Build history of the part. All positions in model axes, mm. A direction names the side the tool comes from. Round coordinates to 2 decimals unless told otherwise and drop trailing zeros. Loops run counter-clockwise (first coordinate to the right, second up) from the corner with the lowest first, then second, coordinate; pieces in that order, holes last. Notation, with made-up numbers: M 85.5,0.5 L 127.5,0.5 A12 cw 127.5,10.5 Z; hole C 62,3.5 d9. An arc over 180 degrees is marked long. Write each question's results on one line, items separated by ' | '. Start each with the question number.
```python
from build123d import *
from build123d.topology import SkipClean

# Parameters (mm, degrees)
CUT_EXTRUDE1_DEPTH  = 11
FILLET1_R           = 8
SKETCH3_R           = 3
CUT_EXTRUDE2_DEPTH  = 3
SKETCH4_R           = 5
CUT_EXTRUDE3_DEPTH  = 4.5
SKETCH5_R           = 25
CUT_EXTRUDE4_DEPTH  = 152.297719745
SKETCH6_R           = 37.5
SKETCH6_R_2         = 35
SKETCH6_R_3         = 27.5
SKETCH6_R_4         = 25
BOSS_EXTRUDE1_DEPTH = 5
CUT_EXTRUDE5_START  = -30
CUT_EXTRUDE5_DEPTH  = 30


# Read off the part's stored shape, not the designer's step: Cut-Extrude5
with BuildPart() as part:
    # Sketch1 → Revolve1 (revolve)
    with BuildSketch(Plane.XY, mode=Mode.PRIVATE) as revolve1_sk:
        Polygon((0, 0), (-50, 0), (-50, 30), (-105, 30), (-105, 40), (-100, 40), (-100, 35), (0, 35), align=None)
    revolve(revolve1_sk.sketch.rotate(Axis((0, 0, 0), (0, 1, 0)), 270), axis=Axis((0, 0, 0), (0, 1, 0)))

    # Sketch2 → Cut-Extrude1 (cut)
    with BuildSketch(Plane.XZ):
        with BuildLine():
            Line((-22.361215932, 21.730762114), (-19.116533878, 16.110807941))
            ThreePointArc((-19.116533878, 16.110807941), (-21.650635095, 12.5), (-23.510635891, 8.5))
            Line((-23.510635891, 8.5), (-30, 8.5))
            ThreePointArc((-30, 8.5), (-38.5, 0), (-30, -8.5))
            Line((-30, -8.5), (-23.510635891, -8.5))
            ThreePointArc((-23.510635891, -8.5), (-21.650635095, -12.5), (-19.116533878, -16.110807941))
            Line((-19.116533878, -16.110807941), (-22.361215932, -21.730762114))
            ThreePointArc((-22.361215932, -21.730762114), (-19.25, -33.341978046), (-7.638784068, -30.230762114))
            Line((-7.638784068, -30.230762114), (-4.394102013, -24.610807941))
            ThreePointArc((-4.394102013, -24.610807941), (0, -25), (4.394102013, -24.610807941))
            Line((4.394102013, -24.610807941), (7.638784068, -30.230762114))
            ThreePointArc((7.638784068, -30.230762114), (19.25, -33.341978046), (22.361215932, -21.730762114))
            Line((22.361215932, -21.730762114), (19.116533878, -16.110807941))
            ThreePointArc((19.116533878, -16.110807941), (21.650635095, -12.5), (23.510635891, -8.5))
            Line((23.510635891, -8.5), (30, -8.5))
            ThreePointArc((30, -8.5), (38.5, 0), (30, 8.5))
            Line((30, 8.5), (23.510635891, 8.5))
            ThreePointArc((23.510635891, 8.5), (21.650635095, 12.5), (19.116533878, 16.110807941))
            Line((19.116533878, 16.110807941), (22.361215932, 21.730762114))
            ThreePointArc((22.361215932, 21.730762114), (19.25, 33.341978046), (7.638784068, 30.230762114))
            Line((7.638784068, 30.230762114), (4.394102013, 24.610807941))
            ThreePointArc((4.394102013, 24.610807941), (0, 25), (-4.394102013, 24.610807941))
            Line((-4.394102013, 24.610807941), (-7.638784068, 30.230762114))
            ThreePointArc((-7.638784068, 30.230762114), (-19.25, 33.341978046), (-22.361215932, 21.730762114))
        make_face()
    extrude(amount=-CUT_EXTRUDE1_DEPTH, mode=Mode.SUBTRACT)

    # Fillet1
    fillet1_edges = [part.edges().sort_by_distance(p)[0] for p in [
        (23.510635891, 5.5, -8.5),
        (19.116533878, 5.5, -16.110807941),
        (-4.394102013, 5.5, -24.610807941),
        (4.394102013, 5.5, -24.610807941),
        (-23.510635891, 5.5, -8.5),
        (-19.116533878, 5.5, -16.110807941),
        (19.116533878, 5.5, 16.110807941),
        (23.510635891, 5.5, 8.5),
        (4.394102013, 5.5, 24.610807941),
        (-4.394102013, 5.5, 24.610807941),
        (-23.510635891, 5.5, 8.5),
        (-19.116533878, 5.5, 16.110807941),
    ]]
    fillet(fillet1_edges, radius=FILLET1_R - 0.0001)  # a hair under: the kernel refuses the full size

    # Sketch3 → Cut-Extrude2 (cut)
    with BuildSketch(Plane.XZ.offset(-11)):
        with Locations(Location((-15, 25.980762114, 0), (0, 0, 270))):
            Circle(SKETCH3_R)
        with Locations(Location((15, 25.980762114, 0), (0, 0, 270))):
            Circle(SKETCH3_R)
        with Locations(Location((30, 0, 0), (0, 0, 270))):
            Circle(SKETCH3_R)
        with Locations(Location((15, -25.980762114, 0), (0, 0, 270))):
            Circle(SKETCH3_R)
        with Locations(Location((-15, -25.980762114, 0), (0, 0, 270))):
            Circle(SKETCH3_R)
        with Locations(Location((-30, 0, 0), (0, 0, 270))):
            Circle(SKETCH3_R)
    extrude(amount=-CUT_EXTRUDE2_DEPTH, mode=Mode.SUBTRACT)

    # Sketch4 → Cut-Extrude3 (cut)
    with BuildSketch(Plane.XZ):
        with Locations(Location((-34.641016151, -20, 0), (0, 0, 270))):
            Circle(SKETCH4_R)
        with Locations(Location((-34.641016151, 20, 0), (0, 0, 270))):
            Circle(SKETCH4_R)
        with Locations(Location((0, 40, 0), (0, 0, 270))):
            Circle(SKETCH4_R)
        with Locations(Location((34.641016151, 20, 0), (0, 0, 270))):
            Circle(SKETCH4_R)
        with Locations(Location((34.641016151, -20, 0), (0, 0, 270))):
            Circle(SKETCH4_R)
        with Locations(Location((0, -40, 0), (0, 0, 270))):
            Circle(SKETCH4_R)
    extrude(amount=-CUT_EXTRUDE3_DEPTH, mode=Mode.SUBTRACT)

    # Sketch5 → Cut-Extrude4 (cut, through all)
    with BuildSketch(Plane.XZ.offset(-11)):
        with Locations(Location((0, 0, 0), (0, 0, 270))):
            Circle(SKETCH5_R)
    extrude(amount=-CUT_EXTRUDE4_DEPTH, mode=Mode.SUBTRACT)

    # Sketch6 → Boss-Extrude1 (add)
    # profile 1 of 2: a face of its own
    with SkipClean():  # the faces are left unmerged after this step: merging them gives an invalid solid
        with BuildSketch(Plane(origin=(0, 35, 0), x_dir=(1, 0, 0), z_dir=(0, 1, 0))):
            with Locations(Location((0, 0, 0), (0, 0, 90))):
                Circle(SKETCH6_R)
            with Locations(Location((0, 0, 0), (0, 0, 270))):
                Circle(SKETCH6_R_2, mode=Mode.SUBTRACT)
        # profile 2 of 2: a face of its own
        with BuildSketch(Plane(origin=(0, 35, 0), x_dir=(1, 0, 0), z_dir=(0, 1, 0))):
            with Locations(Location((0, 0, 0), (0, 0, 90))):
                Circle(SKETCH6_R_3)
            with Locations(Location((0, 0, 0), (0, 0, 270))):
                Circle(SKETCH6_R_4, mode=Mode.SUBTRACT)
        extrude(amount=BOSS_EXTRUDE1_DEPTH)
    add(part.part.scale(1), mode=Mode.REPLACE)  # the faces are merged on a copy

    # Cut-Extrude5 outline → Cut-Extrude5 (cut)
    with BuildSketch(Plane.XZ.offset(CUT_EXTRUDE5_START)):
        with BuildLine():
            Line((7.5, 23.848480035), (7.5, 49.434299833))
            ThreePointArc((7.5, 49.434299833), (0, 50), (-7.5, 49.434299833))
            Line((-7.5, 49.434299833), (-7.5, 23.848480035))
            ThreePointArc((-7.5, 23.848480035), (0, 25), (7.5, 23.848480035))
        make_face()
    extrude(amount=CUT_EXTRUDE5_DEPTH, mode=Mode.SUBTRACT)


solid = part.part
```
Item 1: Mould opens along X. For faces 4 (the flat face through (-23, 0, -12)), 5 (the cylindrical face through (3.949, 5.577, -26.043)) say: released by +X, released by -X, zero draft, split by the parting line, or undercut.
Item 2: Saw through at C-C, the plane y = 32.5. Give the cut face in (x, z).
Item 3: Drill centre lines: line 1 along X through (y, z) = (38.4, 0); line 2 along Y through (x, z) = (6.5, 33.5); line 3 along X through (y, z) = (2.5, -20). Where is each one in solid material? Low to high. Write a range as [from, to].
Item 4: Tool access for faces 1 (the cylindrical face through (24.63, 5.577, 9.543)), 2 (the cylindrical face through (-4.05, 5.58, -26.1)), 3 (the cylindrical face through (24.397, 37.465, -12.69)): list every direction of +Z, -Z, +X, -X, +Y, -Y with a clear straight run to the whole face (end or side of a thin tool).
Item 5: Saw through at B-B, the plane x = -55.5. Give the cut face in (y, z).
Item 6: Saw through at D-D, the plane z = -59. Give the cut face in (x, y).
Item 7: Drop flat-ended pins along their axis: pin 1 (2 mm diameter, centred on x = -17.5, y = 19, fed in from +Z); pin 2 (13 mm diameter, centred on y = 13.5, z = 33.5, fed in from +X); pin 3 (1.1 mm diameter, centred on x = -29.5, y = 4, fed in from -Z); pin 4 (11 mm diameter, centred on x = -2, z = -37.5, fed in from -Y). Give the stop position or say it passes through.
Working result:
1) face 4: zero draft | face 5: undercut
2) outline: C 0,0 d210; hole C 0,-0.01 d49.99
3) line 1: x = [-105, -100], [-37.5, -35], [-27.5, -25], [25, 27.5], [35, 37.5], [100, 105] | line 2: y = [30, 35] | line 3: x = [-45.83, -39.64], [-29.64, -21.39], [21.39, 29.64], [39.64, 45.83]
4) face 1: -Y | face 2: +Z, -Y | face 3: +Y
5) outline: M 30,-89.13 L 40,-89.13 L 40,-83.19 L 35,-83.19 L 35,83.19 L 40,83.19 L 40,89.13 L 30,89.13 Z
6) outline: M -86.86,30 L 86.86,30 L 86.86,40 L 80.74,40 L 80.74,35 L -80.74,35 L -80.74,40 L -86.86,40 Z
7) pin 1: stops at z = 47.2 | pin 2: stops at x = 42.08 | pin 3: stops at z = -40.77 | pin 4: stops at y = 0
